The drawing under review shows one solid part. Ordinate dimensions are in mm from its lowest x, y, z. A direction names the side the tool comes from. Give positions to 0.01 mm unless a question says otherwise; leave off trailing zeros. Write each loop counter-clockwise with the first axis right and the second up, starting at its lowest first coordinate (ties: lowest second). Pieces come first, ordered by that corner, then holes. Notation, with made-up numbers: (78.5, -21.5) -> (105.5, -21.5) arc R14 ccw to (105.5, -16.5) -> close; hole circle Ø3 at (29.25, 14.25). An arc over 180 degrees is marked (long way). Use CSV: the item, a comma, the result in double quotes.
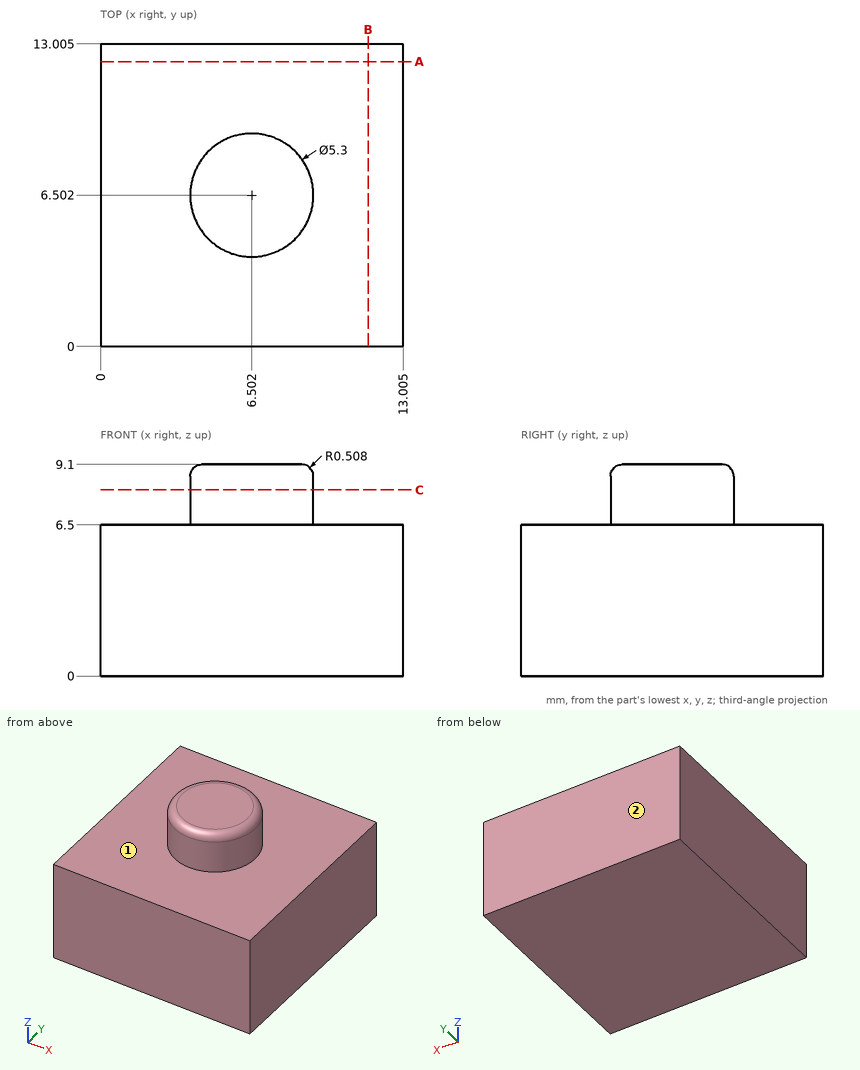
(1) Clearance check with flat-ended pins moving along their axes: pin 1 (1 mm diameter, centred on y = 4.5, z = 8, fed in from -X); pin 2 (4 mm diameter, centred on y = 9, z = 5, fed in from -X). State where each tip first meets the part, or that it passes through.
Established:
pin 1,"stops at x = 4.32"
pin 2,"stops at x = 0"
(2) For line 1 along Z through (x, y) = (1.25, 8); line 2 along Y through (x, z) = (8.5, 7.25) (1 decimal); line 3 along Y through (x, z) = (8, 7) (1 decimal), list the stretches that pass through material, from the lowest coordinate up. Write a range as [from, to].
Established:
line 1,"z = [0, 6.5]"
line 2,"y = [4.8, 8.2]"
line 3,"y = [4.3, 8.7]"
(3) Take a section at A-A (y = 12.25). Write out the cut boundary in (x, z) (1 decimal).
Established:
outline,"(0, 0) -> (13, 0) -> (13, 6.5) -> (0, 6.5) -> close"
(4) Tool access review of the marked faces 1 and 2: name each direction out of +Z, -Z, +X, -X, +Y, -Y from which nothing blocks a thin tool from reaching the whole face with its end or side.
Established:
face 1,"+Z"
face 2,"+Z, -Z, +X, -X, +Y"
(5) Take a section at C-C (z = 8). Write out the cut boundary in (x, y).
Established:
outline,"circle Ø5.3 at (6.5, 6.5)"
